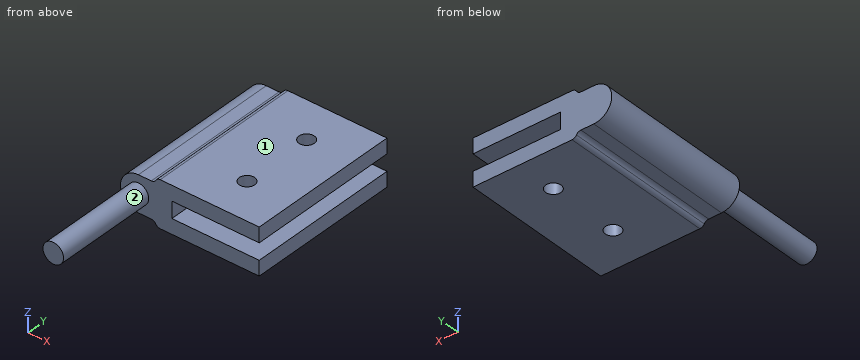
Autodesk Inventor part; units mm, degrees
ref_plane "YZ Plane" through (0, 0, 0) normal (1, 0, 0) x (0, 1, 0)
ref_plane "XZ Plane" through (0, 0, 0) normal (0, 1, 0) x (-1, 0, 0)
ref_plane "XY Plane" through (0, 0, 0) normal (0, 0, 1) x (1, 0, 0)
sketch "Sketch1" plane through (0, 0, 0) normal (0, 1, 0) x (-1, 0, 0)
  line L0 (9.2679, -4.5) -> (-10, -4.5)
  line L1 (-10, 4.5) -> (9.2679, 4.5)
  line L2 (10, -4.5) -> (-10, 4.5) construction
  line L3 (-10, -4.5) -> (10, 4.5) construction
  arc A0 (13.5, -3.5) -> (13.5, 3.5) centre (13.5, 0) ccw
  line L4 (13.5, -3.5) -> (11, -3.5)
  line L5 (13.5, 3.5) -> (11, 3.5)
  line L6 (-10, -1.6) -> (7, -1.6)
  line L7 (7, -1.6) -> (7, 1.6)
  line L8 (7, 1.6) -> (-10, 1.6)
  line L9 (-10, -4.5) -> (-10, -1.6)
  line L10 (-10, 1.6) -> (-10, 4.5)
  line L11 (10, 4.5) -> (10, 4.5)
  line L12 (10, -4.5) -> (10, -4.5)
  arc A1 (11, -3.5) -> (10.134, -4) centre (11, -4.5) ccw
  arc A2 (10.134, 4) -> (11, 3.5) centre (11, 4.5) ccw
  arc A3 (9.2679, -4.5) -> (10.134, -4) centre (9.2679, -3.5) ccw
  arc A4 (10.134, 4) -> (9.2679, 4.5) centre (9.2679, 3.5) ccw
  point P0 (0, 0)
  dimension "d24" = 20
  dimension "d25" = 9
  dimension "d26" = 7
  dimension "d27" = 2.9
  dimension "d28" = 2.9
  dimension "d30" = 1
extrude "Extrusion4" add sketch "Sketch1" along normal blind 30
sketch "Sketch4" plane through (0, 0, 0) normal (0, -1, 0) x (1, 0, 0)
  arc A0 (-13.5, 3.5) -> (-13.5, -3.5) centre (-13.5, 0) ccw
  circle A1 centre (-13.5, 0) radius 2
  point P0 (0, 0)
  dimension "d33" = 4
extrude "Extrusion5" add sketch "Sketch4" along normal blind 20
sketch "Sketch5" plane through (-9.2679, 0, 4.5) normal (0, 0, 1) x (1, 0, 0)
  circle A0 centre (10.2679, 22) radius 1.5
  circle A1 centre (10.2679, 8) radius 1.5
  line L0 (19.2679, 0) -> (19.2679, 30)
  line L1 (0, 30) -> (19.2679, 30)
  line L2 (0, 0) -> (19.2679, 0)
  point P0 (9.2679, 0)
  dimension "d36" = 3
  dimension "d37" = 3
  dimension "d38" = 9
  dimension "d39" = 9
  dimension "d40" = 8
  dimension "d41" = 8
extrude "Extrusion6" cut sketch "Sketch5" against normal blind 20
properties part number "joint male"
Could you check a few things on this model? Use its own coordinates, in mm. Face numbers are marked on the shaded views. A direction names the side the tool comes from. Coordinates: 2 decimals unless noted, no trailing zeros. Write each loop counter-clockwise with the first axis right and the second up, starting at its lowest first coordinate (ties: lowest second). Pieces come first, ordered by that corner, then holes. Notation, with made-up numbers: (55, 13.5) - (81, 13.5) arc R19 cw to (81, 25.5) - close; hole circle Ø5 at (16, 59.25). An arc over 180 degrees is marked (long way). Write item = value, one per line.
1) Please list where these lines run through material, in increasing order: line 1 (Y direction, x = 1, z = -3.75); line 2 (Z direction, x = -3, y = 16); line 3 (Y direction, x = 2, z = 3.25). Write a range as [from, to].
Result set:
line_1 = [0, 6.5], [9.5, 20.5], [23.5, 30]
line_2 = [-4.5, -1.6], [1.6, 4.5]
line_3 = [0, 6.88], [9.12, 20.88], [23.12, 30]
2) Will these pins go through, and if not, where does the flat tip stop? pin 1 Ø2 at (x, y) = (-12.5, 19.5) entering from +Z; pin 2 Ø1.2 at (x, y) = (-12.5, 15) entering from -Z; pin 3 Ø2 at (y, z) = (19, -3) entering from -X.
Result set:
pin_1 = 3.5
pin_2 = -3.5
pin_3 = -16.37
3) Suppose I cut it at D-D on y = 10. Please give me the cut outline in (x, z), plus the area to 3 significant figures.
Result set:
outline = (-13.5, -3.5) - (-11, -3.5) arc R1 cw to (-10.13, -4) arc R1 ccw to (-9.27, -4.5) - (10, -4.5) - (10, -1.6) - (-7, -1.6) - (-7, 1.6) - (10, 1.6) - (10, 4.5) - (-9.27, 4.5) arc R1 ccw to (-10.13, 4) arc R1 cw to (-11, 3.5) - (-13.5, 3.5) arc R3.5 ccw to start
area = 170 mm2
4) Suppose I cut it at B-B on y = 22. Please give me the cut outline in (x, z), plus the area to 3 significant figures.
Result set:
outline = (-13.5, -3.5) - (-11, -3.5) arc R1 cw to (-10.13, -4) arc R1 ccw to (-9.27, -4.5) - (-0.5, -4.5) - (-0.5, -1.6) - (-7, -1.6) - (-7, 1.6) - (-0.5, 1.6) - (-0.5, 4.5) - (-9.27, 4.5) arc R1 ccw to (-10.13, 4) arc R1 cw to (-11, 3.5) - (-13.5, 3.5) arc R3.5 ccw to start; (2.5, -4.5) - (10, -4.5) - (10, -1.6) - (2.5, -1.6) - close; (2.5, 1.6) - (10, 1.6) - (10, 4.5) - (2.5, 4.5) - close
area = 152 mm2
5) Suppose I cut it at C-C on z = 0. Please give me the cut outline in (x, y).
Result set:
outline = (-17, 0) - (-15.5, 0) - (-15.5, -20) - (-11.5, -20) - (-11.5, 0) - (-7, 0) - (-7, 30) - (-17, 30) - close
6) For the marked faces 1 and 2, which set-ups out of +Z, -Z, +X, -X, +Y, -Y let a thin tool reach every point of the face, with its end or its side?
Result set:
face_1 = +Z, +X, -X, +Y, -Y
face_2 = -Y
7) Suppose I cut it at A-A on x = -1. Please give me the cut outline in (y, z).
Result set:
outline = (0, -4.5) - (30, -4.5) - (30, -1.6) - (0, -1.6) - close; (0, 1.6) - (30, 1.6) - (30, 4.5) - (0, 4.5) - close
